For this review, take the finished solid that the model builds, in its own axes (mm). A direction names the side the tool comes from. Round coordinates to 2 decimals unless told otherwise and drop trailing zeros. Order: outer loops, then holes, each group sorted by start corner. A loop starts at its lowest first (then second) coordinate and runs counter-clockwise, first axis right, second up. Notation, with made-up numbers: (23, -9.5) - (37, -9.5) arc R29 cw to (37, 28.5) - close; hole circle Ø2 at (89, 80.5). An arc over 180 degrees is marked (long way). One line per item, written item: value.
```python
from build123d import *

# Parameters (mm, degrees)
BOSS_EXTRUDE1_DEPTH = 10
BOSS_EXTRUDE2_DEPTH = 29


with BuildPart() as part:
    # Sketch1 → Boss-Extrude1 (new body)
    with BuildSketch(Plane.XY):
        Polygon((3.043765375, 8.102399012), (39.923255905, 1.544552589), (108.379559315, 55.783588702), (125.526610048, 30.521909453), (39.211607002, -28.066742617), (10.726491113, -23.001569193), (-3.966827285, -43.324835363), (-23.780494778, -28.999946703), align=None)
    boss_extrude1 = extrude(amount=-BOSS_EXTRUDE1_DEPTH)

    # Sketch2 → Boss-Extrude2 (add)
    with BuildSketch(Plane(origin=(0, 0, -10), x_dir=(-1, 0, 0), z_dir=(0, 0, -1))):
        Polygon((-59.712812316, 17.224138126), (-74.292234429, -4.25481419), (-125.526610048, 30.521909453), (-108.379559315, 55.783588702), align=None)
        Polygon((23.780494778, -28.999946703), (3.966827285, -43.324835363), (-4.420221287, -31.724173356), (15.393446206, -17.399284696), align=None)
    boss_extrude2 = extrude(amount=BOSS_EXTRUDE2_DEPTH)

    # Mirror1: Boss-Extrude1, Boss-Extrude2 across plane
    add(boss_extrude1.mirror(Plane.XY.offset(-39)))
    add(boss_extrude2.mirror(Plane.XY.offset(-39)))


solid = part.part
```
Item 1: Take a section at B-B (x = 57). Write out the cut boundary in (y, z), plus the area to 3 significant figures.
Returned:
outline: (-15.99, -78) - (15.07, -78) - (15.07, -68) - (-15.99, -68) - close; (-15.99, -10) - (15.07, -10) - (15.07, 0) - (-15.99, 0) - close
area: 621 mm^2
Item 2: Take a section at D-D (y = 39). Write out the cut boundary in (x, z).
Returned:
outline: (87.2, -78) - (119.77, -78) - (119.77, 0) - (87.2, 0) - close
Item 3: The part is to be moulded in two halves that separate along X. For faces 1 (the flat face through (51, -1, 0)), 2 (the flat face through (25.17, -25.57, -4.93)), 3 (the flat face through (-13.735, -36.263, -39.546)), say which applies: +X half, -X half, draft (parallel to the pull), parting line (faces both ways), or undercut.
Returned:
face 1: draft
face 2: undercut
face 3: -X half
Item 4: Take a section at A-A (z = -43.5). Write out the cut boundary in (x, y).
Returned:
outline: (-23.78, -29) - (-3.97, -43.32) - (4.42, -31.72) - (-15.39, -17.4) - close; (59.71, 17.22) - (74.29, -4.25) - (125.53, 30.52) - (108.38, 55.78) - close
Item 5: Take a section at C-C (z = -72). Write out the cut boundary in (x, y), plus the area to 3 significant figures.
Returned:
outline: (-23.78, -29) - (-3.97, -43.32) - (10.73, -23) - (39.21, -28.07) - (125.53, 30.52) - (108.38, 55.78) - (39.92, 1.54) - (3.04, 8.1) - close
area: 4,420 mm^2
Item 6: For P1, Ø2, axis at y = 12, z = -62, coming from the +X side; P2, Ø2, axis at y = -19.5, z = -48.5, coming from the +X side; P3, Ø12, axis at x = 55, z = -17, coming from the +Y side, all flat-tipped, find the tip position at first contact; note any pin that passes through.
Returned:
P1: x = 99.71
P2: x = -11.1
P3: y = 18.24
Item 7: Machinability: for faces 4 (the flat face through (30, -7, -10)), 5 (the flat face through (21.23, 4.87, -73.07)), 6 (the flat face through (66.9, 6.635, -39.406)), which of the approach directions +Z, -Z, +X, -X, +Y, -Y give a long, thin tool a straight path to every point of the face, cutting with its end or side? Answer none if there is none.
Returned:
face 4: none
face 5: +Z, -Z, +Y
face 6: -X, -Y
Item 8: Wall thickness on line 1 (Z direction, x = 43, y = -10.5); line 2 (X direction, y = 36.5, z = -61); line 3 (X direction, y = 34.5, z = -36.5): over which ranges is each line inside the solid? List them lowest first.
Returned:
line 1: -78 to -68, -10 to 0
line 2: 84.04 to 121.47
line 3: 81.52 to 122.83
